Design review of the part built by this model. Coordinates are the model's own, in mm. A direction names the side the tool comes from. Coordinates: 2 decimals unless noted, no trailing zeros. Loops run counter-clockwise (first coordinate to the right, second up) from the corner with the lowest first, then second, coordinate; pieces in that order, holes last. Notation, with made-up numbers: (23, -11) -> (38, -11) arc R6 cw to (38, -7) -> close; hole circle Ø5 at (48, 78). An arc over 180 degrees is marked (long way). One line per item, written item: value. Start each with the question number.
1. Insertion check: pin 1 (1 mm diameter, centred on x = 5.5, y = -18.5, fed in from +Z); pin 2 (1.5 mm diameter, centred on y = 21, z = -16, fed in from +X); pin 3 (4 mm diameter, centred on x = 21, z = -3.5, fed in from +Y). Each pin has a flat end and moves straight along its axis. Give the tip position at first contact, or say it passes through.
2. Add section A-A on z = -4.25. Write out the cut boundary in (x, y) (3 decimals), plus the area to 3 significant figures.
3. For probe 1 along X at (y, z) = (-15, -4.5); probe 2 along Z at (x, y) = (9.5, -29); probe 3 along X at (y, z) = (-7, -15.25), list the stretches that pass through material, from the lowest coordinate up.
4. Add section D-D on z = -15. Write out the cut boundary in (x, y) (3 decimals), plus the area to 3 significant figures.
5. Add section B-B on y = -3.5. Write out the cut boundary in (x, z), plus the area to 3 significant figures.
6. Add section C-C on x = -14. Write out the cut boundary in (y, z) (3 decimals).
7. Draft analysis for pull direction X (two halves, no side actions). For faces 3 (the cylindrical face through (-23.52, 0.48, -17.1)), 4 (the flat face through (26.886, 0, -7)), 5 (the flat face through (24.854, 0, -8)), state which applies: pulls with the +X half, pulls with the -X half, needs draft (parallel to the pull), parting line crosses it, or undercut.
8. Machinability: for faces 1 (the flat face through (-23.062, 0, -9)), 2 (the flat face through (1, -3, -18.63)), which of the approach directions +Z, -Z, +X, -X, +Y, -Y give a long, thin tool a straight path to every point of the face, cutting with its end or side? Answer none if there is none.
```python
from build123d import *

# Parameters (mm, degrees)
F1_DEPTH    = 34.52499953
F2_T1_DEPTH = 94.44999906
F2_T3_DEPTH = 77.25000044


# Not quite as in the source:
# - a fillet or chamfer that OpenCascade refuses, or shapes differently, is made with other operations: its cross-section is extruded or revolved along the edge and cut away or added


with BuildPart() as f1:
    # F0 (on Front) → F1 (new body, symmetric)
    with BuildSketch(Plane.XZ):
        Polygon((-24.9640439777, 0), (-24.9640439777, -18.630000078), (26.8859564623, -18.630000078), (26.8859564623, 0), (24.8539564623, 0), (24.8539564623, -16.881729), (-23.0624323377, -16.881729), (-23.0624323377, 0), align=None)
    extrude(amount=F1_DEPTH, both=True)

    # F2: fillet of radius 5.08 on 3 edges, made by hand

    # F2_s2 → F2_t1 (cut)
    with BuildSketch(Plane.XZ.offset(-47.22499953)):
        with BuildLine():
            ThreePointArc((26.8859564623, -13.550000078), (25.3980589107, -17.1421025264), (21.8059564623, -18.630000078))
            Line((21.8059564623, -18.630000078), (26.8859564623, -18.630000078))
            Line((26.8859564623, -18.630000078), (26.8859564623, -13.550000078))
        make_face()
        with BuildLine():
            ThreePointArc((-24.9640439777, -13.550000078), (-23.4761464261, -17.1421025264), (-19.8840439777, -18.630000078))
            Line((-19.8840439777, -18.630000078), (-24.9640439777, -18.630000078))
            Line((-24.9640439777, -18.630000078), (-24.9640439777, -13.550000078))
        make_face()
    extrude(amount=F2_T1_DEPTH, mode=Mode.SUBTRACT)

    # F2_s4 → F2_t3 (cut)
    with BuildSketch(Plane.YZ.offset(-37.6640439777)):
        with BuildLine():
            ThreePointArc((29.44499953, -18.630000078), (33.0371019784, -17.1421025264), (34.52499953, -13.550000078))
            Line((34.52499953, -13.550000078), (34.52499953, -18.630000078))
            Line((34.52499953, -18.630000078), (29.44499953, -18.630000078))
        make_face()
    extrude(amount=F2_T3_DEPTH, mode=Mode.SUBTRACT)


solid = f1.part
```
Worked answers:
1. pin 1: stops at z = -16.88
1. pin 2: stops at x = 26.59
1. pin 3: passes through
2. outline: (-24.964, -34.525) -> (-23.062, -34.525) -> (-23.062, 34.525) -> (-24.964, 34.525) -> close; (24.854, -34.525) -> (26.886, -34.525) -> (26.886, 34.525) -> (24.854, 34.525) -> close
2. area: 272 mm²
3. probe 1: x = -24.96 to -23.06, 24.85 to 26.89
3. probe 2: z = -18.63 to -16.88
3. probe 3: x = -24.67 to -23.06, 24.85 to 26.59
4. outline: (-24.753, -34.525) -> (-23.062, -34.525) -> (-23.062, 34.314) -> (-24.753, 34.314) -> close; (24.854, -34.525) -> (26.675, -34.525) -> (26.675, 34.314) -> (24.854, 34.314) -> close
4. area: 242 mm²
5. outline: (-24.96, -13.55) arc R5.08 ccw to (-19.88, -18.63) -> (21.81, -18.63) arc R5.08 ccw to (26.89, -13.55) -> (26.89, 0) -> (24.85, 0) -> (24.85, -16.88) -> (-23.06, -16.88) -> (-23.06, 0) -> (-24.96, 0) -> close
5. area: 146 mm²
6. outline: (-34.525, -18.63) -> (29.445, -18.63) arc R5.08 ccw to (33.28, -16.882) -> (-34.525, -16.882) -> close
7. face 3: pulls with the -X half
7. face 4: pulls with the +X half
7. face 5: undercut
8. face 1: +Z, +Y, -Y
8. face 2: -Z, +X, -X, +Y, -Y
